from build123d import *

# Parameters (mm, degrees)
SKETCH_2_W                         = 90
SKETCH_2_H                         = 60
SM_BASE_FLANGE_1_DEPTH             = 3
SM_EDGE_FLANGE_1_STRIP_W           = 13.4732
SM_EDGE_FLANGE_1_STRIP_H           = 3
SM_EDGE_FLANGE_1_STRIP_CUT_DEPTH   = 90
SM_EDGE_FLANGE_1_DEPTH             = 90
SM_EDGE_FLANGE_2_STRIP_W           = 13.4732
SM_EDGE_FLANGE_2_STRIP_H           = 3
SM_EDGE_FLANGE_2_STRIP_CUT_DEPTH   = 56.2634
SM_EDGE_FLANGE_2_STRIP_2_W         = 13.4732
SM_EDGE_FLANGE_2_STRIP_2_H         = 3
SM_EDGE_FLANGE_2_STRIP_CUT_2_DEPTH = 56.2634
SM_EDGE_FLANGE_2_DEPTH             = 56.2634
SM_EDGE_FLANGE_2_BEND_DEPTH        = 56.2634
HOLE_WIZARD_M6_1_D                 = 5
FILLET_1_R                         = 30


# Sheet-metal steps are written as plain solids
with BuildPart() as part:
    # Sketch 2 → 基体-法兰1 (new body)
    with BuildSketch(Plane.XY):
        Rectangle(SKETCH_2_W, SKETCH_2_H)
    extrude(amount=-SM_BASE_FLANGE_1_DEPTH)

    # 边线-法兰1 strip (across the edge) → 边线-法兰1 strip cut (cut)
    with BuildSketch(Plane(origin=(45, 30, 0), x_dir=(0, -1, 0), z_dir=(-1, 0, 0))):
        with Locations((-3, -1.5)):
            Rectangle(SM_EDGE_FLANGE_1_STRIP_W, SM_EDGE_FLANGE_1_STRIP_H)
    extrude(amount=SM_EDGE_FLANGE_1_STRIP_CUT_DEPTH, mode=Mode.SUBTRACT)

    # 边线-法兰1 section (across the edge) → 边线-法兰1 (add)
    with BuildSketch(Plane(origin=(45, 30, 0), x_dir=(0, -1, 0), z_dir=(-1, 0, 0))):
        with BuildLine():
            Line((0, 0.7366), (0, 42))
            Line((0, 42), (3, 42))
            Line((3, 42), (3, 0.7366))
            ThreePointArc((3, 0.7366), (3.215745145, 0.215745145), (3.7366, 0))
            Line((3.7366, 0), (3.7366, -3))
            ThreePointArc((3.7366, -3), (1.094424801, -1.905575199), (0, 0.7366))
        make_face()
    extrude(amount=SM_EDGE_FLANGE_1_DEPTH)

    # 边线-法兰2 strip (across the edge) → 边线-法兰2 strip cut (cut)
    with BuildSketch(Plane(origin=(-45, 26.2634, 0), x_dir=(1, 0, 0), z_dir=(0, -1, 0))):
        with Locations((-3, -1.5)):
            Rectangle(SM_EDGE_FLANGE_2_STRIP_W, SM_EDGE_FLANGE_2_STRIP_H)
    extrude(amount=SM_EDGE_FLANGE_2_STRIP_CUT_DEPTH, mode=Mode.SUBTRACT)

    # 边线-法兰2 strip 2 (across the edge) → 边线-法兰2 strip cut 2 (cut)
    with BuildSketch(Plane(origin=(45, -30, 0), x_dir=(-1, 0, 0), z_dir=(0, 1, 0))):
        with Locations((-3, -1.5)):
            Rectangle(SM_EDGE_FLANGE_2_STRIP_2_W, SM_EDGE_FLANGE_2_STRIP_2_H)
    extrude(amount=SM_EDGE_FLANGE_2_STRIP_CUT_2_DEPTH, mode=Mode.SUBTRACT)

    # 边线-法兰2 section (across the edge) → 边线-法兰2 (add)
    with BuildSketch(Plane(origin=(-45, 26.2634, 0), x_dir=(1, 0, 0), z_dir=(0, -1, 0))):
        with BuildLine():
            Line((0, 0.7366), (0, 42))
            Line((0, 42), (3, 42))
            Line((3, 42), (3, 0.7366))
            ThreePointArc((3, 0.7366), (3.215745145, 0.215745145), (3.7366, 0))
            Line((3.7366, 0), (3.7366, -3))
            ThreePointArc((3.7366, -3), (1.094424801, -1.905575199), (0, 0.7366))
        make_face()
    extrude(amount=SM_EDGE_FLANGE_2_DEPTH)

    # 边线-法兰2 section 2 (across the edge) → 边线-法兰2 bend (add)
    with BuildSketch(Plane(origin=(45, -30, 0), x_dir=(-1, 0, 0), z_dir=(0, 1, 0))):
        with BuildLine():
            Line((0, 0.7366), (0, 42))
            Line((0, 42), (3, 42))
            Line((3, 42), (3, 0.7366))
            ThreePointArc((3, 0.7366), (3.215745145, 0.215745145), (3.7366, 0))
            Line((3.7366, 0), (3.7366, -3))
            ThreePointArc((3.7366, -3), (1.094424801, -1.905575199), (0, 0.7366))
        make_face()
    extrude(amount=SM_EDGE_FLANGE_2_BEND_DEPTH)

    # M6 螺纹孔1 (through all)
    with Locations(Plane(origin=(0, 0, -3), x_dir=(-1, 0, 0), z_dir=(0, 0, -1))):
        with Locations((-25.5, 14), (-25.5, -22), (25.5, -22), (25.5, 14)):
            Hole(HOLE_WIZARD_M6_1_D / 2)

    # 圆角1
    fillet_1_edges = [part.edges().sort_by_distance(p)[0] for p in [
        (43.5, -30, 42),
        (-43.5, -30, 42),
    ]]
    fillet(fillet_1_edges, radius=FILLET_1_R)


solid = part.part
Could you check a few things on this model? Use its own coordinates, in mm. A direction names the side the tool comes from. Give positions to 0.01 mm unless a question says otherwise; leave off trailing zeros. Order: outer loops, then holes, each group sorted by start corner. A loop starts at its lowest first (then second) coordinate and runs counter-clockwise, first axis right, second up.
1. Suppose I cut it at A-A (z = 4). List the corners of the cut face in (x, y) for me, plus the area to 3 significant figures.
2. Suppose I cut it at B-B (x = -25.5). List the corners of the cut face in (y, z) for me.
3. Will these pins go through, and if not, where does the flat tip stop? P1, Ø1.5, axis at x = 4, y = -14.5, coming from the +Z side; P2, Ø6, axis at x = 25.5, y = -22, coming from the -Z side.
4. Suppose I cut it at D-D (x = 17.5). List the corners of the cut face in (y, z) for me, plus the area to 3 significant figures.
5. Suppose I cut it at C-C (y = 14). List the corners of the cut face in (x, z) for me.
6. We'd pull the mould along X, two halves only. Please class faces 1 (the cylindrical face through (43.88, -2.26, -1.93)), 2 (the flat face through (-1, -1, 0)), 3 (the flat face through (-44, 13, 42)): pulls with the +X half, pulls with the -X half, needs draft (parallel to the pull), parting line crosses it, or undercut.
7. For faces 4 (the flat face through (44, 26.263, 21)), 5 (the flat face through (-42, -1, 22)), 6 (the flat face through (-44.1, 26.263, -2.2)), which set-ups out of +Z, -Z, +X, -X, +Y, -Y let a thin tool reach every point of the face, with its end or its side?
8. I need wall thicknesses on L1, parallel to X at y = 22, z = 35.5; L2, parallel to Y at x = 25.5, z = -1.15; L3, parallel to Y at x = 25.5, z = -1.7. Which ranges of each line are inside material? Lowest first, please.
Solved:
1. outline: (-45, -30) - (-42, -30) - (-42, 26.26) - (-45, 26.26) - close; (-45, 27) - (45, 27) - (45, 30) - (-45, 30) - close; (42, -30) - (45, -30) - (45, 26.26) - (42, 26.26) - close
1. area: 608 mm2
2. outline: (-30, -3) - (-24.5, -3) - (-24.5, 0) - (-30, 0) - close; (-19.5, -3) - (11.5, -3) - (11.5, 0) - (-19.5, 0) - close; (16.5, -3) - (26.26, -3) arc R3.74 ccw to (30, 0.74) - (30, 42) - (27, 42) - (27, 0.74) arc R0.74 cw to (26.26, 0) - (16.5, 0) - close
3. P1: stops at z = 0
3. P2: stops at z = -3
4. outline: (-30, -3) - (26.26, -3) arc R3.74 ccw to (30, 0.74) - (30, 42) - (27, 42) - (27, 0.74) arc R0.74 cw to (26.26, 0) - (-30, 0) - close
4. area: 303 mm2
5. outline: (-45, 0.74) arc R3.74 ccw to (-41.26, -3) - (-28, -3) - (-28, 0) - (-41.26, 0) arc R0.74 cw to (-42, 0.74) - (-42, 42) - (-45, 42) - close; (-23, -3) - (23, -3) - (23, 0) - (-23, 0) - close; (28, -3) - (41.26, -3) arc R3.74 ccw to (45, 0.74) - (45, 42) - (42, 42) - (42, 0.74) arc R0.74 cw to (41.26, 0) - (28, 0) - close
6. face 1: pulls with the +X half
6. face 2: undercut
6. face 3: needs draft
7. face 4: +Z, +X, -X
7. face 5: +Z, -Y
7. face 6: -Z, -X, -Y
8. L1: x = -45 to -42, 42 to 45
8. L2: y = -30 to -24.5, -19.5 to 11.5, 16.5 to 29.49
8. L3: y = -30 to -24.5, -19.5 to 11.5, 16.5 to 29.1
